from build123d import *

# Parameters (mm, degrees)
F0_W  = 76.2
F0_H  = 76.2
F2_W  = 38.1
F2_H  = 38.1
F4_W  = 38.1
F4_H  = 38.1
F8_D  = 3.81
F10_D = 3.81


with BuildPart() as f3:
    # F0 (on Top) → F3 section 0
    with BuildSketch(Plane.XY):
        Rectangle(F0_W, F0_H)
    # F2 (on offset) → F3 section 1
    with BuildSketch(Plane.XY.offset(38.1)):
        Rectangle(F2_W, F2_H)
    loft()

    # F10 (through all)
    with Locations(Plane.XY.offset(38.1)):
        with Locations((0, 0)):
            Hole(F10_D / 2)


with BuildPart() as f6:
    # F4 (on offset) → F6 section 0
    with BuildSketch(Plane.XY.offset(38.1), mode=Mode.PRIVATE) as f6_s0:
        Rectangle(F4_W, F4_H)
    loft([f6_s0.sketch, Vertex(0, 0, 76.5771791339)])

    # F8 (through all)
    with Locations(Plane(origin=(0, 0, 38.1), x_dir=(1, 0, 0), z_dir=(0, 0, -1))):
        with Locations((0, 0)):
            Hole(F8_D / 2)


solid = f6.part
Build history of the part. All positions in model axes, mm. Round coordinates to 2 decimals unless told otherwise and drop trailing zeros. Loops run counter-clockwise (first coordinate to the right, second up) from the corner with the lowest first, then second, coordinate; pieces in that order, holes last. Notation, with made-up numbers: (24, 84.25) -> (62, 84.25) arc R36 ccw to (62, 120.25) -> close; hole circle Ø2 at (41, -25). An arc over 180 degrees is marked (long way). Use CSV: the item, a comma, the result in double quotes. Start each with the question number.
Q1. Flat gauge pins, fed straight in: pin 1 Ø2 at (x, y) = (11.5, -9.5) entering from +Z; pin 2 Ø12 at (x, z) = (-3.5, 55.5) entering from +Y; pin 3 Ø5 at (x, z) = (-1.5, 52) entering from -Y. Where does each tip first touch, or does it go through?
Q2. Drill centre lines: L1, parallel to Y at x = 1, z = 70.5; L2, parallel to X at y = 1.5, z = 46.5; L3, parallel to Y at x = -1, z = 49. Where is each one in solid material? Low to high.
Q3. Saw through at B-B on x = 0. Give the cut face in (y, z) (3 decimals), and give its area (3 significant figures).
Q4. Saw through at A-A on z = 68. Give the cut face in (x, y) (3 decimals).
Q5. Mould opens along X. For faces 1 (the face through (12.04, -0.27, 52.26)), 2 (the face through (-1.817, -0.572, 56.229)), 3 (the face through (-12.04, 0.27, 52.26)), 4 (the face through (0.27, 12.04, 52.26)) say: +X half, -X half, draft (parallel to the pull), parting line (faces both ways), or undercut.
Q6. Saw through at D-D on z = 52. Give the cut face in (x, y) (3 decimals).
Solutions:
1,pin 1,"stops at z = 55.37"
1,pin 2,"stops at y = 13.41"
1,pin 3,"stops at y = -13.41"
2,L1,"y = -3.01 to -1.62, 1.62 to 3.01"
2,L2,"x = -14.89 to -1.17, 1.17 to 14.89"
2,L3,"y = -13.65 to -1.62, 1.62 to 13.65"
3,outline,"(-19.05, 38.1) -> (-1.905, 38.1) -> (-1.905, 72.729) -> close; (1.905, 38.1) -> (19.05, 38.1) -> (1.905, 72.729) -> close"
3,area,"594 mm^2"
4,outline,"(-4.247, -4.247) -> (4.247, -4.247) -> (4.247, 4.247) -> (-4.247, 4.247) -> close; hole circle Ø3.81 at (0, 0)"
5,face 1,"+X half"
5,face 2,"undercut"
5,face 3,"-X half"
5,face 4,"draft"
6,outline,"(-12.168, -12.168) -> (12.168, -12.168) -> (12.168, 12.168) -> (-12.168, 12.168) -> close; hole circle Ø3.81 at (0, 0)"
